Answer from the drawing. Dimensions are ordinates in mm from the lowest x, y and z of the part. Give positions to 0.01 mm unless a question says otherwise; leave off trailing zeros. Order: outer loops, then holes, each group sorted by start corner. A loop starts at its lowest first (then second) coordinate and runs counter-clockwise, first axis right, second up.
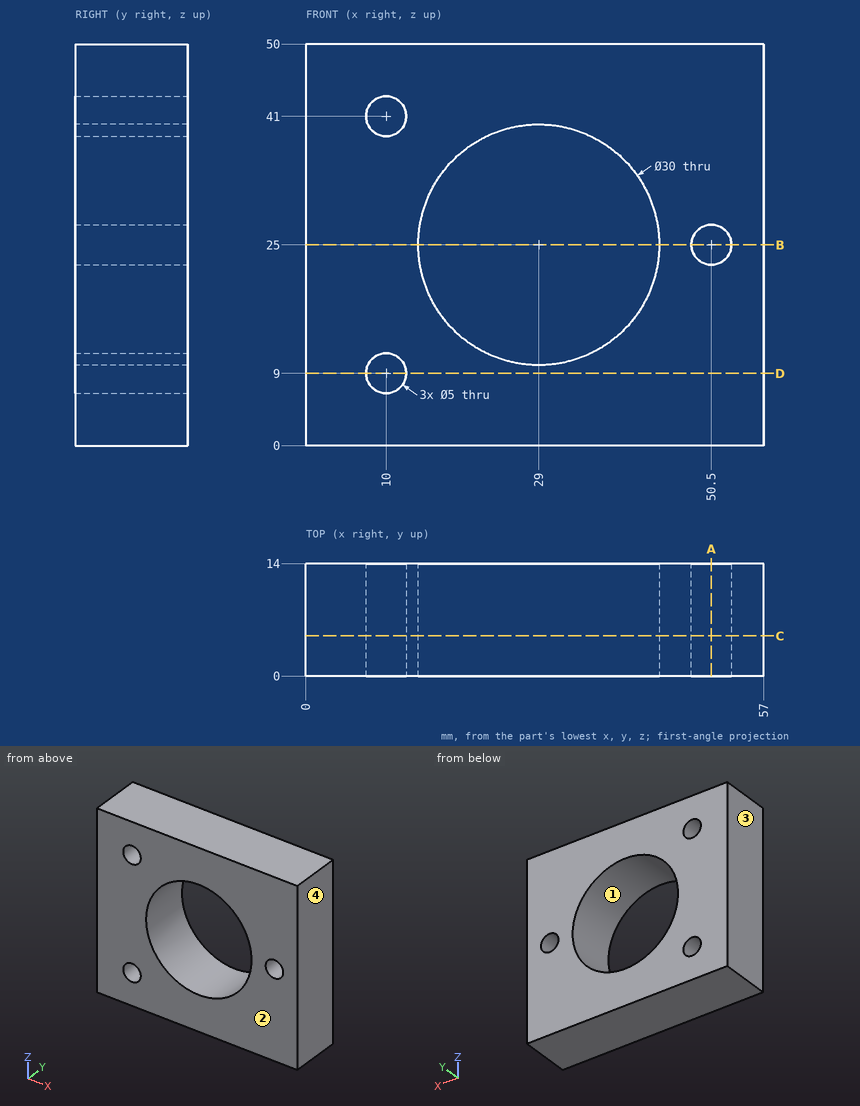
1. The part is cut by section B-B (z = 25). Write down the section's boundary in (x, y), then the cut area to 3 significant figures.
Findings below:
outline: (0, 0) - (14, 0) - (14, 14) - (0, 14) - close; (44, 0) - (48, 0) - (48, 14) - (44, 14) - close; (53, 0) - (57, 0) - (57, 14) - (53, 14) - close
area: 308 mm2
2. The part is cut by section D-D (z = 9). Write down the section's boundary in (x, y).
Findings below:
outline: (0, 0) - (7.5, 0) - (7.5, 14) - (0, 14) - close; (12.5, 0) - (57, 0) - (57, 14) - (12.5, 14) - close
3. The part is cut by section C-C (y = 5). Write down the section's boundary in (x, z).
Findings below:
outline: (0, 0) - (57, 0) - (57, 50) - (0, 50) - close; hole circle Ø5 at (10, 9); hole circle Ø5 at (10, 41); hole circle Ø30 at (29, 25); hole circle Ø5 at (50.5, 25)
4. The part is cut by section A-A (x = 50.5). Write down the section's boundary in (y, z).
Findings below:
outline: (0, 0) - (14, 0) - (14, 22.5) - (0, 22.5) - close; (0, 27.5) - (14, 27.5) - (14, 50) - (0, 50) - close
5. Straight lines are drawn through the part: probe 1 along Z at (x, y) = (10, 9.75); probe 2 along Z at (x, y) = (50.5, 7); probe 3 along Z at (x, y) = (29, 3.25). For each, find the intervals that lie inside material, in ascending order.
Findings below:
probe 1: z = 0 to 6.5, 11.5 to 38.5, 43.5 to 50
probe 2: z = 0 to 22.5, 27.5 to 50
probe 3: z = 0 to 10, 40 to 50
6. The mould has two halves that part along X. Classify the marked faces 1, 2, 3 and 4: pulls with the +X half, pulls with the -X half, needs draft (parallel to the pull), parting line crosses it, or undercut.
Findings below:
face 1: undercut
face 2: needs draft
face 3: pulls with the -X half
face 4: pulls with the +X half
